Design review of the part built by this model. Coordinates are the model's own, in mm. Round coordinates to 2 decimals unless told otherwise and drop trailing zeros. Order: outer loops, then holes, each group sorted by start corner. A loop starts at its lowest first (then second) coordinate and runs counter-clockwise, first axis right, second up. Notation, with made-up numbers: (84, 43) - (127, 43) arc R20 cw to (127, 79) - close; hole circle Ø5 at (80, 66.5). An arc over 180 degrees is marked (long way). Answer as a JSON object with one key per item and string values. Group by question number.
from build123d import *

# Parameters (mm, degrees)
SKETCH_1_R      = 55
SKETCH_1_R_2    = 1.5
EXTRUDE_2_DEPTH = 3


with BuildPart() as part:
    # 草图1 → 凸台-拉伸2 (new body)
    with BuildSketch(Plane(origin=(0, 0, 0), x_dir=(1, 0, 0), z_dir=(0, 1, 0))):
        with BuildLine():
            Line((-60, 70), (60, 70))
            ThreePointArc((60, 70), (130, 0), (60, -70))
            Line((60, -70), (-60, -70))
            ThreePointArc((-60, -70), (-130, 0), (-60, 70))
        make_face()
        with Locations((-60, 0)):
            Circle(SKETCH_1_R, mode=Mode.SUBTRACT)
        with Locations((60, 0)):
            Circle(SKETCH_1_R, mode=Mode.SUBTRACT)
        with Locations((-122, 0)):
            Circle(SKETCH_1_R_2, mode=Mode.SUBTRACT)
        with Locations((122, 0)):
            Circle(SKETCH_1_R_2, mode=Mode.SUBTRACT)
        with Locations((-30, 60)):
            Circle(SKETCH_1_R_2, mode=Mode.SUBTRACT)
        with Locations((30, 60)):
            Circle(SKETCH_1_R_2, mode=Mode.SUBTRACT)
        with Locations((30, -60)):
            Circle(SKETCH_1_R_2, mode=Mode.SUBTRACT)
        with Locations((-30, -60)):
            Circle(SKETCH_1_R_2, mode=Mode.SUBTRACT)
        with Locations((-49.58110934, 59.088465181)):
            Circle(SKETCH_1_R_2, mode=Mode.SUBTRACT)
        with Locations((-116.381557247, -20.5212086)):
            Circle(SKETCH_1_R_2, mode=Mode.SUBTRACT)
        with Locations((-14.037333413, -38.567256581)):
            Circle(SKETCH_1_R_2, mode=Mode.SUBTRACT)
        with Locations((14.037333413, -38.567256581)):
            Circle(SKETCH_1_R_2, mode=Mode.SUBTRACT)
        with Locations((116.381557247, -20.5212086)):
            Circle(SKETCH_1_R_2, mode=Mode.SUBTRACT)
        with Locations((49.58110934, 59.088465181)):
            Circle(SKETCH_1_R_2, mode=Mode.SUBTRACT)
    extrude(amount=EXTRUDE_2_DEPTH)


solid = part.part
1. To check wall thickness, follow line 1 (X direction, y = 0.65, z = 0); line 2 (X direction, y = 1.5, z = -60); line 3 (X direction, y = 0.2, z = -11). State the ranges of each line that lie inside material, in increasing order. Write a range as from..to.
2. Take a section at C-C, the plane y = 1.55. Count the separate pieces of the cut face and the enclosed holes in it, then the cut area to 3 significant figures.
3. Clearance check with flat-ended pins moving along their axes: P1, Ø1.8, axis at x = -30, z = 60, coming from the -Y side; P2, Ø1, axis at y = 2.5, z = 6, coming from the +X side. State where each tip first meets the part, or that it passes through.
4. Take a section at D-D, the plane x = 54.5. Give the boundary of the cut face in (y, z), then the cut area to 3 significant figures.
5. Take a section at B-B, the plane z = 10.5. Give the boundary of the cut face in (x, y).
6. Mouldability with a two-part tool opening along X and no side actions: class faces 1 (the cylindrical face through (48.077, 1.479, 53.692)), 2 (the flat face through (2, 0, -1)), 3 (the cylindrical face through (129.983, 1.479, -1.539)) as pulls with the +X half, pulls with the -X half, needs draft (parallel to the pull), parting line crosses it, or undercut.
7. Take a section at A-A, the plane x = -18. Give the boundary of the cut face in (y, z), then the cut area to 3 significant figures.
Response values:
{
 "1": {"line 1": "-130..-123.5, -120.5..-115, -5..5, 115..120.5, 123.5..130", "line 2": "-96.06..-50.77, -48.39..-31.5, -28.5..28.5, 31.5..48.39, 50.77..96.06", "line 3": "-129.13..-113.89, -6.11..6.11, 113.89..129.13"},
 "2": {"separate pieces": "1", "enclosed holes": "14", "area": "13,100 mm2"},
 "3": {"P1": "through", "P2": "x = 129.78"},
 "4": {"outline": "(0, -70) - (3, -70) - (3, -54.72) - (0, -54.72) - close; (0, 54.72) - (3, 54.72) - (3, 70) - (0, 70) - close", "area": "91.7 mm2"},
 "5": {"outline": "(-129.21, 0) - (-113.99, 0) - (-113.99, 3) - (-129.21, 3) - close; (-6.01, 0) - (6.01, 0) - (6.01, 3) - (-6.01, 3) - close; (113.99, 0) - (129.21, 0) - (129.21, 3) - (113.99, 3) - close"},
 "6": {"face 1": "undercut", "face 2": "needs draft", "face 3": "pulls with the +X half"},
 "7": {"outline": "(0, -70) - (3, -70) - (3, -35.51) - (0, -35.51) - close; (0, 35.51) - (3, 35.51) - (3, 70) - (0, 70) - close", "area": "207 mm2"}
}
